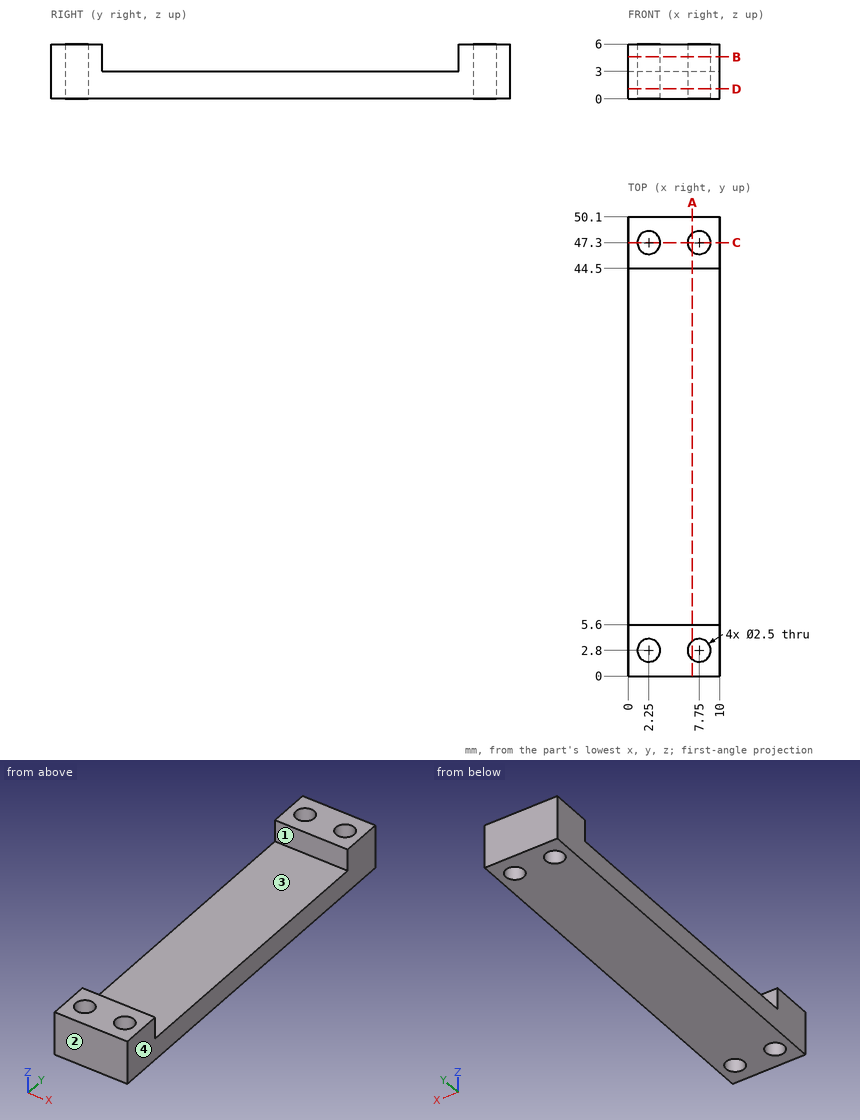
The drawing under review shows one solid part. Ordinate dimensions are in mm from its lowest x, y, z. Round coordinates to 2 decimals unless told otherwise and drop trailing zeros. Order: outer loops, then holes, each group sorted by start corner. A loop starts at its lowest first (then second) coordinate and runs counter-clockwise, first axis right, second up. Notation, with made-up numbers: M 6,78 L 30,78 A28 cw 30,113 Z; hole C 63,-11.75 d6. An arc over 180 degrees is marked long. Answer as CSV lines item,"result". Start each with the question number.
1) Add section C-C (y = 47.3). Give the boundary of the cut face in (x, z), then the cut area to 3 significant figures.
2) Add section D-D (z = 1.1). Give the boundary of the cut face in (x, y), then the cut area to 3 significant figures.
3) Add section A-A (x = 7). Give the boundary of the cut face in (y, z).
4) Wall thickness on line 1 along Y through (x, z) = (7.75, 1.25); line 2 along Y through (x, z) = (1.75, 4.8); line 3 along Y through (x, z) = (5.75, 3.55): over which ranges is each line inside the solid? List them lowest first. Write a range as [from, to].
5) The part is to be moulded in two halves that separate along Y. For the marked faces 1, 2, 3 and 4, say which applies: +Y half, -Y half, draft (parallel to the pull), parting line (faces both ways), or undercut.
6) Add section B-B (z = 4.6). Give the boundary of the cut face in (x, y), then the cut area to 3 significant figures.
7) For pin 1 Ø2 at (x, y) = (6.5, 26) entering from +Z; pin 2 Ø0.9 at (x, z) = (4, 4.5) entering from -Y; pin 3 Ø2 at (x, y) = (7.75, 47.3) entering from -Z, all flat-tipped, find the tip position at first contact; note any pin that passes through.
Resolved:
1,outline,"M 0,0 L 1,0 L 1,6 L 0,6 Z; M 3.5,0 L 6.5,0 L 6.5,6 L 3.5,6 Z; M 9,0 L 10,0 L 10,6 L 9,6 Z"
1,area,"30.0 mm^2"
2,outline,"M 0,0 L 10,0 L 10,50.1 L 0,50.1 Z; hole C 2.25,2.8 d2.5; hole C 2.25,47.3 d2.5; hole C 7.75,2.8 d2.5; hole C 7.75,47.3 d2.5"
2,area,"481 mm^2"
3,outline,"M 0,0 L 1.8,0 L 1.8,6 L 0,6 Z; M 3.8,0 L 46.3,0 L 46.3,6 L 44.5,6 L 44.5,3 L 5.6,3 L 5.6,6 L 3.8,6 Z; M 48.3,0 L 50.1,0 L 50.1,6 L 48.3,6 Z"
4,line 1,"[0, 1.55], [4.05, 46.05], [48.55, 50.1]"
4,line 2,"[0, 1.65], [3.95, 5.6], [44.5, 46.15], [48.45, 50.1]"
4,line 3,"[0, 5.6], [44.5, 50.1]"
5,face 1,"undercut"
5,face 2,"-Y half"
5,face 3,"undercut"
5,face 4,"draft"
6,outline,"M 0,0 L 10,0 L 10,5.6 L 0,5.6 Z; M 0,44.5 L 10,44.5 L 10,50.1 L 0,50.1 Z; hole C 2.25,2.8 d2.5; hole C 2.25,47.3 d2.5; hole C 7.75,2.8 d2.5; hole C 7.75,47.3 d2.5"
6,area,"92.4 mm^2"
7,pin 1,"z = 3"
7,pin 2,"y = 0"
7,pin 3,"through"
